Can you work these out from the model? Positions are in its coordinate system, mm. A direction names the side the tool comes from. Give positions to 0.01 mm unless a question says otherwise; leave off trailing zeros. Loops run counter-clockwise (first coordinate to the right, second up) from the corner with the lowest first, then second, coordinate; pieces in that order, holes last. Notation, with made-up numbers: M 56.25,49 L 102.25,49 A17 cw 102.25,81 Z; hole C -24,10 d10. An arc over 180 degrees is marked long. Answer as a JSON object with one key per item and string values.
Autodesk Inventor part; units mm, degrees
ref_plane "YZ Plane" through (0, 0, 0) normal (1, 0, 0) x (0, 1, 0)
ref_plane "XZ Plane" through (0, 0, 0) normal (0, 1, 0) x (-1, 0, 0)
ref_plane "XY Plane" through (0, 0, 0) normal (0, 0, 1) x (1, 0, 0)
sketch "Sketch1" plane through (0, 0, 0) normal (0, 0, 1) x (1, 0, 0)
  line L0 (-8, 0) -> (8, 0) construction
  line L1 (-8, -4) -> (8, -4)
  line L2 (8, 4) -> (-8, 4)
  arc A0 (-8, 4) -> (-8, -4) centre (-8, 0) ccw
  arc A1 (8, -4) -> (8, 4) centre (8, 0) ccw
  point P0 (0, 0)
  dimension "d0" = 16
  dimension "d1" = 4
extrude "Extrusion1" add sketch "Sketch1" along normal blind 8
chamfer "Chamfer1" distance 0.5 angle 45 8 edges at (0, 4, 8) (-12, 0, 8) (0, -4, 8) (12, 0, 8) (0, 4, 0) (-12, 0, 0) (0, -4, 0) (12, 0, 0)
sketch "Sketch2" plane through (0, 0, 8) normal (0, 0, 1) x (1, 0, 0)
  point P0 (0, 0)
hole "Hole1" at (0, 0, 8) direction (0, 0, -1) diameter 4 end through all counterbore diameter 6 counterbore depth 2
properties part number "Slider" material "Steel"
1) Will these pins go through, and if not, where does the flat tip stop? pin 1 Ø2 at (y, z) = (-2.5, 6.5) entering from +X; pin 2 Ø1.5 at (y, z) = (-1, 6.5) entering from +X.
Answer list:
{"pin 1": "x = 11.71", "pin 2": "x = 11.99"}
2) If we mould it in two halves opening along Y, with no side actions, what happens to faces 1 (the conical face through (-11.64, 0.08, 0.14)), 2 (the flat face through (-0.2, 2.4, 0)), 3 (the flat face through (2, -1, 6))? For each: +Y half, -Y half, draft (parallel to the pull), parting line (faces both ways), or undercut.
Answer list:
{"face 1": "parting line", "face 2": "draft", "face 3": "undercut"}
3) Suppose I cut it at B-B, the plane y = 0. Write out the boundary of the cut face in (x, z), and give its area (4 significant figures).
Answer list:
{"outline": "M -12,0.5 L -11.5,0 L -2,0 L -2,6 L -3,6 L -3,8 L -11.5,8 L -12,7.5 Z; M 2,0 L 11.5,0 L 12,0.5 L 12,7.5 L 11.5,8 L 3,8 L 3,6 L 2,6 Z", "area": "155.5 mm^2"}
4) For faces 4 (the flat face through (0, -4, 4)), 5 (the cylindrical face through (0, 3, 7)), which set-ups out of +Z, -Z, +X, -X, +Y, -Y let a thin tool reach every point of the face, with its end or its side?
Answer list:
{"face 4": "+Z, -Z, +X, -X, -Y", "face 5": "+Z"}
5) Please list where these lines run through material, in increasing order: line 1 along Y through (x, z) = (0, 1.5); line 2 along X through (y, z) = (0, 6.5); line 3 along X through (y, z) = (0, 2.3). Write a range as from..to.
Answer list:
{"line 1": "-4..-2, 2..4", "line 2": "-12..-3, 3..12", "line 3": "-12..-2, 2..12"}
6) Suppose I cut it at C-C, the plane z = 0.75. Write out the boundary of the cut face in (x, y).
Answer list:
{"outline": "M -8,-4 L 8,-4 A4 ccw 8,4 L -8,4 A4 ccw Z; hole C 0,0 d4"}
7) Suppose I cut it at A-A, the plane x = 0. Write out the boundary of the cut face in (y, z).
Answer list:
{"outline": "M -4,0.5 L -3.5,0 L -2,0 L -2,6 L -3,6 L -3,8 L -3.5,8 L -4,7.5 Z; M 2,0 L 3.5,0 L 4,0.5 L 4,7.5 L 3.5,8 L 3,8 L 3,6 L 2,6 Z"}
